Work out the finished part from the listing and answer in its coordinate system (mm). Coordinates: 2 decimals unless noted, no trailing zeros. Loops run counter-clockwise (first coordinate to the right, second up) from the corner with the lowest first, then second, coordinate; pieces in that order, holes last. Notation, with made-up numbers: (61, 46) -> (115, 46) arc R22 ccw to (115, 84) -> close; hole circle Ø4 at (76, 20). An arc over 180 degrees is marked (long way). Use a Markdown table: item, result.
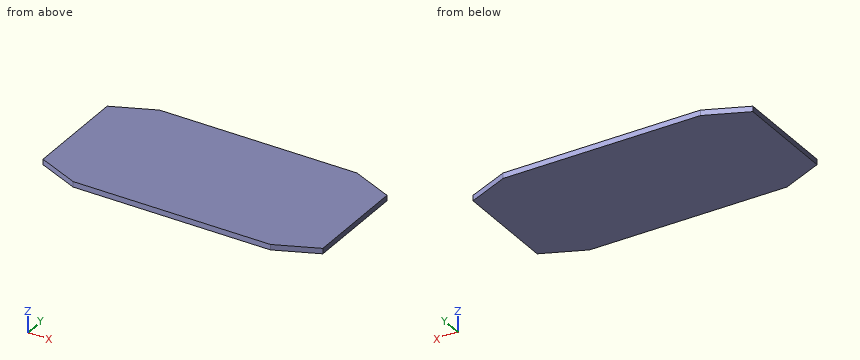
from build123d import *

# Parameters (mm, degrees)
BOX004_W               = 20
BOX004_H               = 10
BOX004_DEPTH           = 10
BOX004_PLACEMENT_ANGLE = 156.5
BOX006_W               = 20
BOX006_H               = 10
BOX006_DEPTH           = 10
BOX006_PLACEMENT_ANGLE = 23.5
BOX007_W               = 20
BOX007_H               = 10
BOX007_DEPTH           = 10
BOX007_PLACEMENT_ANGLE = -23.5
BOX005_W               = 20
BOX005_H               = 10
BOX005_DEPTH           = 10
BOX005_PLACEMENT_ANGLE = 203.5
BOX001_W               = 108.5
BOX001_H               = 54
BOX001_DEPTH           = 2.1


with BuildPart() as cube004:
    # Box004 → Box004 (new body)
    with BuildSketch(Plane.XY):
        with Locations((10, 5)):
            Rectangle(BOX004_W, BOX004_H)
    extrude(amount=BOX004_DEPTH)


with BuildPart() as cube004_1:
    # Box004 placement: moved
    add(cube004.part.moved(Location((16, 0, 0))).rotate(Axis((16, 0, 0), (0, 0, 1)), BOX004_PLACEMENT_ANGLE))


with BuildPart() as cube006:
    # Box006 → Box006 (new body)
    with BuildSketch(Plane.XY):
        with Locations((10, 5)):
            Rectangle(BOX006_W, BOX006_H)
    extrude(amount=BOX006_DEPTH)


with BuildPart() as cube006_1:
    # Box006 placement: moved
    add(cube006.part.moved(Location((94.5, -10.035, 0))).rotate(Axis((94.5, -10.035, 0), (0, 0, 1)), BOX006_PLACEMENT_ANGLE))


with BuildPart() as cube007:
    # Box007 → Box007 (new body)
    with BuildSketch(Plane.XY):
        with Locations((10, 5)):
            Rectangle(BOX007_W, BOX007_H)
    extrude(amount=BOX007_DEPTH)


with BuildPart() as cube007_1:
    # Box007 placement: moved
    add(cube007.part.moved(Location((92.5, 54, 0))).rotate(Axis((92.5, 54, 0), (0, 0, 1)), BOX007_PLACEMENT_ANGLE))


with BuildPart() as cube005:
    # Box005 → Box005 (new body)
    with BuildSketch(Plane.XY):
        with Locations((10, 5)):
            Rectangle(BOX005_W, BOX005_H)
    extrude(amount=BOX005_DEPTH)


with BuildPart() as cube005_1:
    # Box005 placement: moved
    add(cube005.part.moved(Location((14, 64.0348, 0))).rotate(Axis((14, 64.0348, 0), (0, 0, 1)), BOX005_PLACEMENT_ANGLE))


with BuildPart() as obj1:
    # Box001 → Box001 (new body)
    with BuildSketch(Plane.XY):
        with Locations((54.25, 27)):
            Rectangle(BOX001_W, BOX001_H)
    extrude(amount=BOX001_DEPTH)

    # Cut001: cut Cube005
    add(cube005_1.part, mode=Mode.SUBTRACT)

    # Cut002: cut Cube007
    add(cube007_1.part, mode=Mode.SUBTRACT)

    # Cut003: cut Cube006
    add(cube006_1.part, mode=Mode.SUBTRACT)

    # Cut004: cut Cube004
    add(cube004_1.part, mode=Mode.SUBTRACT)


with BuildPart() as obj1_1:
    # Cut004 placement: moved
    add(obj1.part.moved(Location((-36.55, -13.7, 20))))


solid = obj1_1.part
Q1. Section B-B on x = 57 is taken. Determine the outline of the cut face in (y, z).
Solved:
| item | result |
|---|---|
| outline | (-13.24, 20) -> (39.84, 20) -> (39.84, 22.1) -> (-13.24, 22.1) -> close |
Q2. Section A-A on z = 20.9 is taken. Determine the outline of the cut face in (x, y), and give its area (3 significant figures).
Solved:
| item | result |
|---|---|
| outline | (-36.55, -6.74) -> (-20.55, -13.7) -> (55.95, -13.7) -> (71.95, -6.74) -> (71.95, 33.34) -> (55.95, 40.3) -> (-20.55, 40.3) -> (-36.55, 33.34) -> close |
| area | 5,640 mm² |
Q3. Section C-C on y = 36.5 is taken. Determine the outline of the cut face in (x, z).
Solved:
| item | result |
|---|---|
| outline | (-29.29, 20) -> (64.69, 20) -> (64.69, 22.1) -> (-29.29, 22.1) -> close |
Q4. Consider line 1 (X direction, y = 35, z = 21.3); line 2 (Y direction, x = 64, z = 21.2); line 3 (X direction, y = 33.5, z = 21.65). Determine where each line is inside the solid, lowest interval first. Write a range as [from, to].
Solved:
| item | result |
|---|---|
| line 1 | [-32.74, 68.14] |
| line 2 | [-10.2, 36.8] |
| line 3 | [-36.19, 71.59] |
